Build history of the part. All positions in model axes, mm. Give positions to 0.01 mm unless a question says otherwise; leave off trailing zeros. Order: outer loops, then holes, each group sorted by start corner. A loop starts at its lowest first (then second) coordinate and runs counter-clockwise, first axis right, second up. Notation, with made-up numbers: (76.25, -23) -> (120.25, -23) arc R19 cw to (120.25, -4) -> close; hole circle Ø8 at (16.25, -2.75). An arc over 180 degrees is marked (long way). One line per question, with ' | ' between items. Start each with the question number.
(1) Cut at B-B (x = -33). Give the cut face in (y, z), then the cut area to 3 significant figures.
(2) Cut at A-A (x = -65). Give the cut face in (y, z), then the cut area to 3 significant figures.
(3) Cut at C-C (z = -40). Give the cut face in (x, y), then the cut area to 3 significant figures.
(4) Drill centre lines: L1, parallel to X at y = -0.8, z = 60.5; L2, parallel to Z at x = -65, y = -0.6; L3, parallel to X at y = -0.4, z = 39. Where is each one in solid material? Low to high. Write a range as from..to.
(5) Cut at D-D (y = -0.7). Give the number of separate pieces and of enclosed holes in the cut face, then the cut area to 3 significant figures.
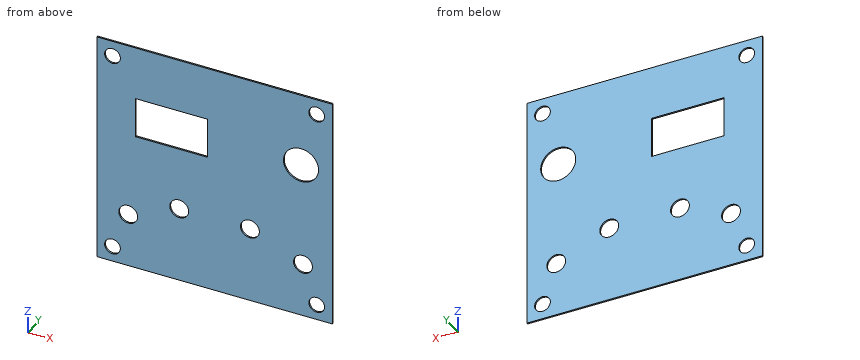
from build123d import *

# Parameters (mm, degrees)
F0_R     = 5
F0_R_2   = 6
F0_W     = 46
F0_H     = 26
F0_R_3   = 11.167495
F1_DEPTH = 1


with BuildPart() as f1:
    # F0 (on Front) → F1 (new body)
    with BuildSketch(Plane.XZ):
        Polygon((75, -75), (75, 75), (-75, 75), (-75, 15), (-75, 0), (-75, -75), align=None)
        with Locations((-65, -65)):
            Circle(F0_R, mode=Mode.SUBTRACT)
        with Locations((-55, -40)):
            Circle(F0_R_2, mode=Mode.SUBTRACT)
        with Locations((-22.511177, -26.278466)):
            Circle(F0_R_2, mode=Mode.SUBTRACT)
        with Locations((65, -65)):
            Circle(F0_R, mode=Mode.SUBTRACT)
        with Locations((56.25, -40)):
            Circle(F0_R_2, mode=Mode.SUBTRACT)
        with Locations((22.511177, -26.278466)):
            Circle(F0_R_2, mode=Mode.SUBTRACT)
        with Locations((-27.41893, 27.41893)):
            Rectangle(F0_W, F0_H, mode=Mode.SUBTRACT)
        with Locations((-65, 65)):
            Circle(F0_R, mode=Mode.SUBTRACT)
        with Locations((55, 27.41893)):
            Circle(F0_R_3, mode=Mode.SUBTRACT)
        with Locations((65, 65)):
            Circle(F0_R, mode=Mode.SUBTRACT)
    extrude(amount=F1_DEPTH)


solid = f1.part
Result set:
1) outline: (-1, -75) -> (0, -75) -> (0, 14.42) -> (-1, 14.42) -> close; (-1, 40.42) -> (0, 40.42) -> (0, 75) -> (-1, 75) -> close | area: 124 mm2
2) outline: (-1, -75) -> (0, -75) -> (0, -70) -> (-1, -70) -> close; (-1, -60) -> (0, -60) -> (0, 60) -> (-1, 60) -> close; (-1, 70) -> (0, 70) -> (0, 75) -> (-1, 75) -> close | area: 130 mm2
3) outline: (-75, -1) -> (-61, -1) -> (-61, 0) -> (-75, 0) -> close; (-49, -1) -> (50.25, -1) -> (50.25, 0) -> (-49, 0) -> close; (62.25, -1) -> (75, -1) -> (75, 0) -> (62.25, 0) -> close | area: 126 mm2
4) L1: x = -75..-67.18, -62.82..62.82, 67.18..75 | L2: z = -75..-70, -60..60, 70..75 | L3: x = -75..-50.42, -4.42..75
5) separate pieces: 1 | enclosed holes: 10 | area: 20,100 mm2
